Geometry: final body of the model. Coordinates: model frame, mm. Face numbers are marked on the shaded views. A direction names the side the tool comes from. Coordinates: 2 decimals unless noted, no trailing zeros. Loops run counter-clockwise (first coordinate to the right, second up) from the corner with the lowest first, then second, coordinate; pieces in that order, holes last. Notation, with made-up numbers: (22, 28) - (79, 28) arc R20 ccw to (79, 62) - close; hole circle Ø9 at (58.25, 77.5). An arc over 180 degrees is marked (long way). Put each result on its own line as item: value. Start each with the question number.
1) Contact query for flat-ended pins moving along their axis: pin 1 Ø7 at (x, z) = (-1.5, -0.5) entering from +Y; pin 2 Ø4 at (x, y) = (-5.5, 20) entering from +Z; pin 3 Ø5 at (x, y) = (11.5, 12.5) entering from +Z; pin 4 Ø11 at (x, z) = (0, 0) entering from -Y. Output: stop coordinate, or through.
2) Section A-A on x = 0. Output: boundary loops of the cut face in (y, z) (3 decimals), and give its area (3 significant figures).
3) Section D-D on z = -9.5. Output: boundary loops of the cut face in (x, y) (3 decimals).
4) Reachability of the marked faces 1 and 2 from +Z, -Z, +X, -X, +Y, -Y: full face, straight path, thin tool, end or side. Return the list, or none.
5) Section B-B on z = 0. Output: boundary loops of the cut face in (x, y), and give its area (3 significant figures).
6) Draft query along Z for the marked faces 3, 4 and 5. Return one class per face: +Z half, -Z half, draft (parallel to the pull), parting line (faces both ways), or undercut.
7) Section C-C on y = 17.25. Output: boundary loops of the cut face in (x, z), and give its area (3 significant figures).
8) Material intervals for line 1 along Y through (x, z) = (0, -9) (3 decimals); line 2 along Z through (x, y) = (5, 11); line 3 along X through (y, z) = (14, -6), sorted ascending. Write a range as from..to.
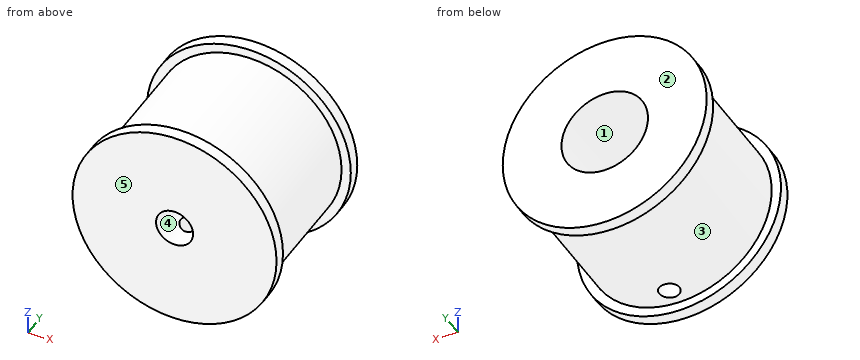
```python
from build123d import *

# Parameters (mm, degrees)
CROQUIS1_R              = 15
CROQUIS1_R_2            = 3
SALIENTE_EXTRUIR1_DEPTH = 25
CROQUIS2_R              = 16.5
CROQUIS2_R_2            = 3
SALIENTE_EXTRUIR2_DEPTH = 2
CROQUIS3_R              = 16.5
CROQUIS3_R_2            = 3
SALIENTE_EXTRUIR3_DEPTH = 2
CORTAR_EXTRUIR1_REACH   = 18.5
CROQUIS4_R              = 1.625
CROQUIS5_R              = 7
CORTAR_EXTRUIR2_DEPTH   = 16


with BuildPart() as part:
    # Croquis1 → Saliente-Extruir1 (new body)
    with BuildSketch(Plane(origin=(0, 0, 0), x_dir=(1, 0, 0), z_dir=(0, 1, 0))):
        Circle(CROQUIS1_R)
        Circle(CROQUIS1_R_2, mode=Mode.SUBTRACT)
    extrude(amount=SALIENTE_EXTRUIR1_DEPTH)

    # Croquis2 → Saliente-Extruir2 (add)
    with BuildSketch(Plane.XZ):
        Circle(CROQUIS2_R)
        Circle(CROQUIS2_R_2, mode=Mode.SUBTRACT)
    extrude(amount=-SALIENTE_EXTRUIR2_DEPTH)

    # Croquis3 → Saliente-Extruir3 (add)
    with BuildSketch(Plane(origin=(0, 25, 0), x_dir=(1, 0, 0), z_dir=(0, 1, 0))):
        Circle(CROQUIS3_R)
        Circle(CROQUIS3_R_2, mode=Mode.SUBTRACT)
    extrude(amount=-SALIENTE_EXTRUIR3_DEPTH)

    # Croquis4 → Cortar-Extruir1 (cut, up to next)
    with BuildSketch(Plane.XY, mode=Mode.PRIVATE) as cortar_extruir1_sk1:
        with Locations((0, 5)):
            Circle(CROQUIS4_R)
    cortar_extruir1_tool1 = extrude(cortar_extruir1_sk1.sketch, amount=-CORTAR_EXTRUIR1_REACH, mode=Mode.PRIVATE) & part.part
    add(cortar_extruir1_tool1.solids().sort_by_distance((0, 5, 0))[0], mode=Mode.SUBTRACT)

    # Croquis5 → Cortar-Extruir2 (cut)
    with BuildSketch(Plane(origin=(0, 25, 0), x_dir=(1, 0, 0), z_dir=(0, 1, 0))):
        Circle(CROQUIS5_R)
    extrude(amount=-CORTAR_EXTRUIR2_DEPTH, mode=Mode.SUBTRACT)


solid = part.part
```
Answer block:
1. pin 1: stops at y = 9
1. pin 2: stops at z = 14.59
1. pin 3: stops at z = 12
1. pin 4: stops at y = 0
2. outline: (0, -16.5) - (2, -16.5) - (2, -15) - (3.375, -15) - (3.375, -3) - (0, -3) - close; (0, 3) - (9, 3) - (9, 7) - (25, 7) - (25, 16.5) - (23, 16.5) - (23, 15) - (2, 15) - (2, 16.5) - (0, 16.5) - close; (6.625, -15) - (23, -15) - (23, -16.5) - (25, -16.5) - (25, -7) - (9, -7) - (9, -3) - (6.625, -3) - close
2. area: 445 mm²
3. outline: (-13.491, 0) - (13.491, 0) - (13.491, 2) - (11.608, 2) - (11.608, 23) - (13.491, 23) - (13.491, 25) - (-13.491, 25) - (-13.491, 23) - (-11.608, 23) - (-11.608, 2) - (-13.491, 2) - close; hole circle Ø3.25 at (0, 5)
4. face 1: +Y
4. face 2: +Z, -Z, +X, -X, +Y
5. outline: (-16.5, 0) - (-3, 0) - (-3, 9) - (-7, 9) - (-7, 25) - (-16.5, 25) - (-16.5, 23) - (-15, 23) - (-15, 2) - (-16.5, 2) - close; (3, 0) - (16.5, 0) - (16.5, 2) - (15, 2) - (15, 23) - (16.5, 23) - (16.5, 25) - (7, 25) - (7, 9) - (3, 9) - close
5. area: 484 mm²
6. face 3: parting line
6. face 4: undercut
6. face 5: draft
7. outline: circle Ø30 at (0, 0); hole circle Ø14 at (0, 0)
7. area: 553 mm²
8. line 1: y = 0..3.375, 6.625..25
8. line 2: z = -14.14..-4.9, 4.9..14.14
8. line 3: x = -13.75..-3.61, 3.61..13.75
